```python
from build123d import *

# Parameters (mm, degrees)
F0_R     = 57.5
F1_DEPTH = 15
F2_DEPTH = 15
F4_COUNT = 5
F6_DEPTH = 3


with BuildPart() as f1:
    # F0 (on Top) → F1 (new body)
    with BuildSketch(Plane.XY):
        Circle(F0_R)
        with BuildLine():
            ThreePointArc((-25.8787150819, 45.6786832747), (26.4349906204, 45.3590263443), (52.5, 0))
            ThreePointArc((52.5, 0), (-24.9083328879, -46.2149862355), (-28.8647601045, 43.8528861548))
            ThreePointArc((-28.8647601045, 43.8528861548), (-27.386956798, 44.7906753393), (-25.8787150819, 45.6786832747))
        make_face(mode=Mode.SUBTRACT)
    extrude(amount=F1_DEPTH)



with BuildPart() as f1b:
    # F0 (on Top) → F1, piece 2 (new body)
    with BuildSketch(Plane.XY):
        with BuildLine():
            ThreePointArc((3, 0), (1, 2.8284271247), (-2.3333333333, 1.8856180832))
            ThreePointArc((-2.3333333333, 1.8856180832), (-2.8284271247, 1), (-3, 0))
            ThreePointArc((-3, 0), (0, -3), (3, 0))
        make_face()
    extrude(amount=F1_DEPTH)


with BuildPart() as f1_1:
    add(f1.part)

    add(f1b.part)  # F2 merges F1b
    # F0 (on Top) → F2 (join)
    with BuildSketch(Plane.XY):
        with BuildLine():
            add(Edge.make_bspline(
                [(-2.3333333333, 1.8856180832), (-10.9416758466, 6.9247769231), (-29.1664290337, 16.1295933501), (-26.623576941, 36.0633998347), (-25.8787150819, 45.6786832747)],
                knots=[0, 0, 0, 0, 0.5034367583, 1, 1, 1, 1], degree=3))
            ThreePointArc((-25.8787150819, 45.6786832747), (-27.386956798, 44.7906753393), (-28.8647601045, 43.8528861548))
            add(Edge.make_bspline(
                [(-3, 0), (-12.803393035, 5.0838333397), (-31.7879164967, 14.9257102522), (-29.8275065593, 34.4356080017), (-28.8647601045, 43.8528861548)],
                knots=[0, 0, 0, 0, 0.5163354868, 1, 1, 1, 1], degree=3))
            ThreePointArc((-3, 0), (-2.8284271247, 1), (-2.3333333333, 1.8856180832))
        make_face()
    extrude(amount=F2_DEPTH)

    # F4: F1 ×5 about axis
    f4_axis = Axis((0, 0, 5.5775735527), (0, 0, -1))


with BuildPart() as f1_2:
    add(f1_1.part)
    for i in range(1, F4_COUNT):
        add(f1_1.part.rotate(f4_axis, i * 360 / F4_COUNT))

    # F5 (on face) → F6 (join)
    with BuildSketch(Plane.XY.offset(15)):
        with BuildLine():
            Line((1.6583123952, 2.5), (-1.6583123952, 2.5))
            ThreePointArc((-1.6583123952, 2.5), (-2.0193254295, 2.2186312919), (-2.3333333333, 1.8856180832))
            ThreePointArc((-2.3333333333, 1.8856180832), (-2.8284271247, 1), (-3, 0))
            ThreePointArc((-3, 0), (-2.8760308636, -0.8534907567), (-2.5143690188, -1.6364438388))
            ThreePointArc((-2.5143690188, -1.6364438388), (-1.8250885652, -2.3809770535), (-0.9270509831, -2.8531695489))
            ThreePointArc((-0.9270509831, -2.8531695489), (-0.0770244674, -2.9990110422), (0.7793678195, -2.8969959962))
            ThreePointArc((0.7793678195, -2.8969959962), (1.700460359, -2.4715247455), (2.4270509831, -1.7633557569))
            ThreePointArc((2.4270509831, -1.7633557569), (2.8284271247, -1), (2.9960448209, -0.1539981522))
            ThreePointArc((2.9960448209, -0.1539981522), (2.8760308636, 0.8534907567), (2.4270509831, 1.7633557569))
            ThreePointArc((2.4270509831, 1.7633557569), (2.0756227182, 2.1660540925), (1.6583123952, 2.5))
        make_face()
    extrude(amount=F6_DEPTH)


solid = f1_2.part
```
For this review, take the finished solid that the model builds, in its own axes (mm). A direction names the side the tool comes from. Round coordinates to 2 decimals unless told otherwise and drop trailing zeros. Put each result on its own line as item: value.
Q1. Insertion check: pin 1 Ø2 at (x, z) = (5.5, 15) entering from -Y; pin 2 Ø3.5 at (x, z) = (0.5, 16.5) entering from +Y; pin 3 Ø3 at (x, z) = (11, 10.5) entering from +Y; pin 4 Ø12 at (x, y) = (27, -37.5) entering from +Z. Each pin has a flat end and moves straight along its axis. Give the tip position at first contact, or say it passes through.
Solved:
pin 1: stops at y = -57.32
pin 2: stops at y = 57.5
pin 3: stops at y = 56.71
pin 4: passes through
Q2. Mouldability with a two-part tool opening along X and no side actions: class faces 3 (the face through (-12.465, -56.133, 7.395)), 4 (the face through (1, 4, 15)), 5 (the face through (-33.8, -40.17, 7.4)) as released by +X, released by -X, zero draft, split by the parting line, or undercut.
Solved:
face 3: split by the parting line
face 4: zero draft
face 5: undercut
Q3. Machinability: for faces 1 (the face through (0, 0, 18)), 2 (the face through (0, 2.5, 16)), which of the approach directions +Z, -Z, +X, -X, +Y, -Y give a long, thin tool a straight path to every point of the face, cutting with its end or side? Answer none if there is none.
Solved:
face 1: +Z, +X, -X, +Y, -Y
face 2: +Z, +X, -X, +Y
Q4. We need section A-A (x = 10). Count the separate pieces of the cut face and the enclosed holes in it, and give its area (3 significant figures).
Solved:
separate pieces: 5
enclosed holes: 0
area: 487 mm2
Q5. Wall thickness on probe 1 along Y at (x, z) = (-18, 3); probe 2 along Y at (x, z) = (36.5, 13.5); probe 3 along X at (y, z) = (21, 9.5): over which ranges is each line inside the solid? List them lowest first.
Solved:
probe 1: y = -54.61 to -49.32, -17.22 to -14.16, 8.64 to 11.86, 49.32 to 54.61
probe 2: y = -44.43 to -37.74, -5.57 to -1.41, 37.74 to 44.43
probe 3: x = -53.53 to -48.12, -28.22 to -24.98, 3.05 to 5.8, 48.12 to 53.53
